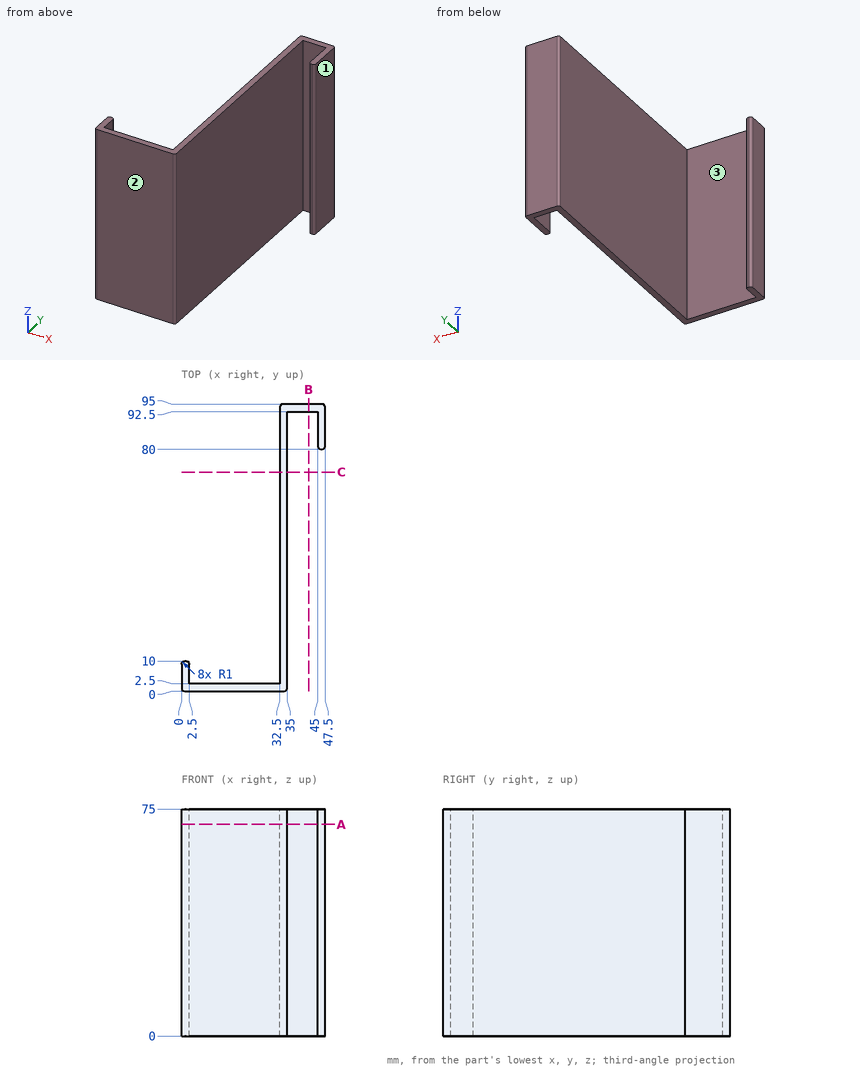
The figure shows three views and two pictorial views of one solid part (mm, origin at its lowest corner). Answer the questions. Give positions to 0.01 mm unless a question says otherwise; leave off trailing zeros. Write each loop counter-clockwise with the first axis right and the second up, starting at its lowest first coordinate (ties: lowest second). Pieces come first, ordered by that corner, then holes. Notation, with made-up numbers: (-24.5, -0.75) - (-4.5, -0.75) arc R27 ccw to (-4.5, 36.25) - close; hole circle Ø6 at (84.5, 32). An arc over 180 degrees is marked (long way). Return JSON: item names as keys, results as strings.
Q1. A cutting plane is placed at A-A, the plane z = 70. Determine the outline of the cut face in (x, y).
Reply:
{"outline": "(0, 1) arc R1 ccw to (1, 0) - (34, 0) arc R1 ccw to (35, 1) - (35, 92.5) - (45, 92.5) - (45, 81) arc R1 ccw to (46, 80) - (46.5, 80) arc R1 ccw to (47.5, 81) - (47.5, 94) arc R1 ccw to (46.5, 95) - (33.5, 95) arc R1 ccw to (32.5, 94) - (32.5, 2.5) - (2.5, 2.5) - (2.5, 9) arc R1 ccw to (1.5, 10) - (1, 10) arc R1 ccw to (0, 9) - close"}
Q2. Consider line 1 along X through (y, z) = (89.5, 6); line 2 along X through (y, z) = (57, 56); line 3 along Y through (x, z) = (19, 60). Determine where each line is inside the solid, lowest interval first. Write a range as [from, to].
Reply:
{"line 1": "[32.5, 35], [45, 47.5]", "line 2": "[32.5, 35]", "line 3": "[0, 2.5]"}
Q3. For a pull along X with two mould halves and no side action, classify the marked faces 1, 2 and 3 as released by +X, released by -X, zero draft, split by the parting line, or undercut.
Reply:
{"face 1": "released by +X", "face 2": "zero draft", "face 3": "undercut"}
Q4. A cutting plane is placed at C-C, the plane y = 72.5. Determine the outline of the cut face in (x, z).
Reply:
{"outline": "(32.5, 0) - (35, 0) - (35, 75) - (32.5, 75) - close"}
Q5. A cutting plane is placed at B-B, the plane x = 42. Determine the outline of the cut face in (y, z), and give its area (4 significant figures).
Reply:
{"outline": "(92.5, 0) - (95, 0) - (95, 75) - (92.5, 75) - close", "area": "187.5 mm²"}
Q6. Given P1, Ø8, axis at y = 80.5, z = 35, coming from the -X side; P2, Ø15, axis at x = 18.5, z = 34.5, coming from the +Y side; P3, Ø6, axis at x = 5, z = 21.5, coming from the +Y side, each flat-ended and moving along its own axis, determine where each tip first touches the part or whether it passes through.
Reply:
{"P1": "x = 32.5", "P2": "y = 2.5", "P3": "y = 9.87"}
